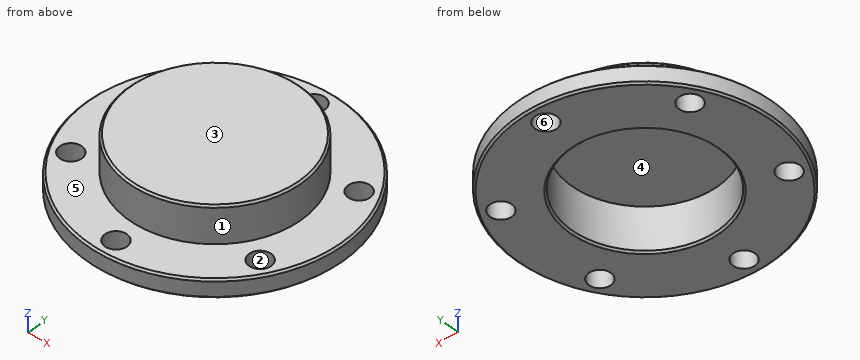
```python
from build123d import *

# Parameters (mm, degrees)
SKETCH_1_R          = 35
EXTRUDE_1_DEPTH     = 5
SKETCH_2_R          = 23.5
EXTRUDE_2_DEPTH     = 10
SKETCH_3_R          = 20
CUT_EXTRUDE_1_DEPTH = 12
SKETCH_4_R          = 3
CUT_EXTRUDE_2_DEPTH = 12
CHAMFER_1_SIZE      = 0.5


with BuildPart() as part:
    # 草图1 → 拉伸1 (new body)
    with BuildSketch(Plane.XY):
        Circle(SKETCH_1_R)
    extrude(amount=EXTRUDE_1_DEPTH)

    # 草图2 → 拉伸2 (add)
    with BuildSketch(Plane.XY.offset(5)):
        Circle(SKETCH_2_R)
    extrude(amount=EXTRUDE_2_DEPTH)

    # 草图3 → 切除-拉伸1 (cut)
    with BuildSketch(Plane(origin=(0, 0, 0), x_dir=(-1, 0, 0), z_dir=(0, 0, -1))):
        Circle(SKETCH_3_R)
    extrude(amount=-CUT_EXTRUDE_1_DEPTH, mode=Mode.SUBTRACT)

    # 草图4 → 切除-拉伸2 (cut)
    with BuildSketch(Plane.XY.offset(5)):
        with Locations((25.980762114, 15)):
            Circle(SKETCH_4_R)
        with Locations((0, 30)):
            Circle(SKETCH_4_R)
        with Locations((25.980762114, -15)):
            Circle(SKETCH_4_R)
        with Locations((0, -30)):
            Circle(SKETCH_4_R)
        with Locations((-25.980762114, -15)):
            Circle(SKETCH_4_R)
        with Locations((-25.980762114, 15)):
            Circle(SKETCH_4_R)
    extrude(amount=-CUT_EXTRUDE_2_DEPTH, mode=Mode.SUBTRACT)

    # 倒角1
    chamfer_1_edges = [part.edges().sort_by_distance(p)[0] for p in [
        (20, 0, 0),
        (-35, 0, 0),
        (-35, 0, 5),
        (-23.5, 0, 15),
    ]]
    chamfer(chamfer_1_edges, length=CHAMFER_1_SIZE)


solid = part.part
```
Can you work these out from the model? Positions are in its coordinate system, mm. Face numbers are marked on the shaded views. A direction names the side the tool comes from. Coordinates: 2 decimals unless noted, no trailing zeros. Order: outer loops, then holes, each group sorted by start corner. A loop starts at its lowest first (then second) coordinate and runs counter-clockwise, first axis right, second up.
1. If we section it at D-D (y = 15): Give the number of separate pieces and of enclosed holes in the cut face, then the cut area to 3 significant figures.
2. Thinking about a two-plate mould opening in X: for the marked faces 1, 2 and 3, which applies, +X half, -X half, draft (parallel to the pull), parting line (faces both ways), or undercut?
3. I need wall thicknesses on line 1 (Y direction, x = 0, z = 4.5); line 2 (X direction, y = -13, z = 3.5); line 3 (Y direction, x = 0, z = 6.75). Which ranges of each line are inside material? Lowest first, please.
4. For the marked faces 4, 5 and 6, which set-ups out of +Z, -Z, +X, -X, +Y, -Y let a thin tool reach every point of the face, with its end or its side?
5. If we section it at C-C (y = 0): Please give me the cut outline in (x, z).
6. If we section it at A-A (x = 0): Please give me the cut outline in (y, z), then the cut area to 3 significant figures.
7. If we section it at B-B (z = 2.25): Please give me the cut outline in (x, y).
8. I'm going to push flat-ended pins straight in: pin 1 (3 mm diameter, centred on y = 14, z = 6, fed in from +X); pin 2 (3 mm diameter, centred on y = 5, z = 12, fed in from -X); pin 3 (4 mm diameter, centred on y = 4, z = 10, fed in from +X); pin 4 (12 mm diameter, centred on x = 22, y = 2.5, fed in from -Z). Where does each tip first touch, or does it pass through?
Entries:
1. separate pieces: 3
1. enclosed holes: 0
1. area: 299 mm2
2. face 1: parting line
2. face 2: undercut
2. face 3: draft
3. line 1: y = -35 to -33, -27 to -20, 20 to 27, 33 to 35
3. line 2: x = -32.5 to -28.22, -23.74 to -15.2, 15.2 to 23.74, 28.22 to 32.5
3. line 3: y = -23.5 to -20, 20 to 23.5
4. face 4: -Z
4. face 5: +Z
4. face 6: +Z, -Z
5. outline: (-35, 0.5) - (-34.5, 0) - (-20.5, 0) - (-20, 0.5) - (-20, 12) - (20, 12) - (20, 0.5) - (20.5, 0) - (34.5, 0) - (35, 0.5) - (35, 4.5) - (34.5, 5) - (23.5, 5) - (23.5, 14.5) - (23, 15) - (-23, 15) - (-23.5, 14.5) - (-23.5, 5) - (-34.5, 5) - (-35, 4.5) - close
6. outline: (-35, 0.5) - (-34.5, 0) - (-33, 0) - (-33, 5) - (-34.5, 5) - (-35, 4.5) - close; (-27, 0) - (-20.5, 0) - (-20, 0.5) - (-20, 12) - (20, 12) - (20, 0.5) - (20.5, 0) - (27, 0) - (27, 5) - (23.5, 5) - (23.5, 14.5) - (23, 15) - (-23, 15) - (-23.5, 14.5) - (-23.5, 5) - (-27, 5) - close; (33, 0) - (34.5, 0) - (35, 0.5) - (35, 4.5) - (34.5, 5) - (33, 5) - close
6. area: 279 mm2
7. outline: circle Ø70 at (0, 0); hole circle Ø6 at (-25.98, -15); hole circle Ø6 at (-25.98, 15); hole circle Ø40 at (0, 0); hole circle Ø6 at (0, -30); hole circle Ø6 at (0, 30); hole circle Ø6 at (25.98, -15); hole circle Ø6 at (25.98, 15)
8. pin 1: stops at x = 32.2
8. pin 2: stops at x = -23.24
8. pin 3: stops at x = 23.41
8. pin 4: stops at z = 0
